Design review of the part built by this model. Coordinates are the model's own, in mm. A direction names the side the tool comes from. Give positions to 0.01 mm unless a question says otherwise; leave off trailing zeros. Write each loop counter-clockwise with the first axis right and the second up, starting at its lowest first coordinate (ties: lowest second). Pieces come first, ordered by that corner, then holes. Notation, with made-up numbers: (74.25, 53) -> (78.25, 53) arc R12 cw to (78.25, 70) -> close; hole circle Ø10 at (53, 3.5). An arc over 180 degrees is marked (long way). Answer as a JSON object with one key per item and string values.
```python
from build123d import *

# Parameters (mm, degrees)
SKETCH1_W            = 40
SKETCH1_H            = 40
BOSS_EXTRUDE1_DEPTH  = 2
EXTRUDE_THIN1_START  = 2
SKETCH1_3_W          = 14
SKETCH1_3_H          = 1
EXTRUDE_THIN1_DEPTH  = 11.2
SKETCH3_R            = 1.5
CUT_EXTRUDE1_DEPTH   = 13.2
LPATTERN1_COUNT      = 2
LPATTERN1_PITCH      = 32
LPATTERN1_COUNT_DIR2 = 2
LPATTERN1_PITCH_DIR2 = 32


with BuildPart() as part:
    # Sketch1 → Boss-Extrude1 (new body)
    with BuildSketch(Plane.XY):
        with Locations((21, 22.483732861)):
            Rectangle(SKETCH1_W, SKETCH1_H)
    extrude(amount=BOSS_EXTRUDE1_DEPTH)

    # Sketch1<3> → Extrude-Thin1 (add)
    with BuildSketch(Plane.XY.offset(EXTRUDE_THIN1_START)):
        with Locations((34, 9.604785493)):
            Rectangle(SKETCH1_3_W, SKETCH1_3_H)
        with Locations((34, 12.320574966)):
            Rectangle(SKETCH1_3_W, SKETCH1_3_H)
        with Locations((34, 15.03636444)):
            Rectangle(SKETCH1_3_W, SKETCH1_3_H)
        with Locations((34, 17.752153914)):
            Rectangle(SKETCH1_3_W, SKETCH1_3_H)
        with Locations((34, 20.467943387)):
            Rectangle(SKETCH1_3_W, SKETCH1_3_H)
        with Locations((34, 23.183732861)):
            Rectangle(SKETCH1_3_W, SKETCH1_3_H)
        with Locations((8, 9.604785493)):
            Rectangle(SKETCH1_3_W, SKETCH1_3_H)
        with Locations((8, 12.320574966)):
            Rectangle(SKETCH1_3_W, SKETCH1_3_H)
        with Locations((8, 15.03636444)):
            Rectangle(SKETCH1_3_W, SKETCH1_3_H)
        with Locations((8, 17.752153914)):
            Rectangle(SKETCH1_3_W, SKETCH1_3_H)
        with Locations((8, 20.467943387)):
            Rectangle(SKETCH1_3_W, SKETCH1_3_H)
        with Locations((8, 23.183732861)):
            Rectangle(SKETCH1_3_W, SKETCH1_3_H)
    extrude(amount=EXTRUDE_THIN1_DEPTH)

    # Sketch3 → Cut-Extrude1 (cut)
    with BuildSketch(Plane(origin=(0, 0, 0), x_dir=(-1, 0, 0), z_dir=(0, 0, -1))):
        with Locations((-37, 6.483732861)):
            Circle(SKETCH3_R)
    cut_extrude1 = extrude(amount=-CUT_EXTRUDE1_DEPTH, mode=Mode.SUBTRACT)

    # LPattern1: Cut-Extrude1 2 × 2
    with Locations(*[(-i * LPATTERN1_PITCH, j * LPATTERN1_PITCH_DIR2, 0) for i in range(LPATTERN1_COUNT) for j in range(LPATTERN1_COUNT_DIR2) if (i, j) != (0, 0)]):
        add(cut_extrude1, mode=Mode.SUBTRACT)


solid = part.part
```
(1) We need section A-A, the plane y = 7.5. State the section outline as (x, z) points, then the cut area to 3 significant figures.
Here are the results:
{"outline": "(1, 0) -> (3.9, 0) -> (3.9, 2) -> (1, 2) -> close; (6.1, 0) -> (35.9, 0) -> (35.9, 2) -> (6.1, 2) -> close; (38.1, 0) -> (41, 0) -> (41, 2) -> (38.1, 2) -> close", "area": "71.2 mm²"}
(2) The part is to be moulded in two halves that separate along Y. For faces 4 (the flat face through (15, 15, 8)), 5 (the flat face through (34, 19.968, 8)), say which applies: +Y half, -Y half, draft (parallel to the pull), parting line (faces both ways), or undercut.
Here are the results:
{"face 4": "draft", "face 5": "undercut"}
(3) We need section B-B, the plane x = 5. Give the number of separate pieces and of enclosed holes in the cut face, then the cut area to 3 significant figures.
Here are the results:
{"separate pieces": "3", "enclosed holes": "0", "area": "135 mm²"}
(4) We need section D-D, the plane x = 31.5. State the section outline as (y, z) points, then the cut area to 3 significant figures.
Here are the results:
{"outline": "(2.48, 0) -> (42.48, 0) -> (42.48, 2) -> (23.68, 2) -> (23.68, 13.2) -> (22.68, 13.2) -> (22.68, 2) -> (20.97, 2) -> (20.97, 13.2) -> (19.97, 13.2) -> (19.97, 2) -> (18.25, 2) -> (18.25, 13.2) -> (17.25, 13.2) -> (17.25, 2) -> (15.54, 2) -> (15.54, 13.2) -> (14.54, 13.2) -> (14.54, 2) -> (12.82, 2) -> (12.82, 13.2) -> (11.82, 13.2) -> (11.82, 2) -> (10.1, 2) -> (10.1, 13.2) -> (9.1, 13.2) -> (9.1, 2) -> (2.48, 2) -> close", "area": "147 mm²"}
(5) For faces 1 (the flat face through (1, 18, 4)), 2 (the flat face through (27, 23, 8)), 3 (the flat face through (8, 22.684, 8)), list the 3-axis set-ups (+Z, -Z, +X, -X, +Y, -Y) from which the entire face can be reached by the end or side of a thin tool; tool diameter is ignored.
Here are the results:
{"face 1": "+Z, -Z, -X, +Y, -Y", "face 2": "+Z, +Y, -Y", "face 3": "+Z, +X, -X"}
(6) For line 1 along Y through (x, z) = (37, 1.1); line 2 along Y through (x, z) = (9.5, 11.75); line 3 along Z through (x, y) = (29, 27), list the stretches that pass through material, from the lowest coordinate up.
Here are the results:
{"line 1": "y = 2.48 to 4.98, 7.98 to 36.98, 39.98 to 42.48", "line 2": "y = 9.1 to 10.1, 11.82 to 12.82, 14.54 to 15.54, 17.25 to 18.25, 19.97 to 20.97, 22.68 to 23.68", "line 3": "z = 0 to 2"}
(7) Clearance check with flat-ended pins moving along their axes: pin 1 (1.8 mm diameter, centred on x = 5, y = 38.48, fed in from -Z); pin 2 (5.5 mm diameter, centred on x = 33.5, z = 7, fed in from +Y); pin 3 (5 mm diameter, centred on x = 5, y = 6.48, fed in from +Z); pin 4 (4 mm diameter, centred on x = 34.5, z = 5, fed in from -Y). State where each tip first meets the part, or that it passes through.
Here are the results:
{"pin 1": "passes through", "pin 2": "stops at y = 23.68", "pin 3": "stops at z = 2", "pin 4": "stops at y = 9.1"}
